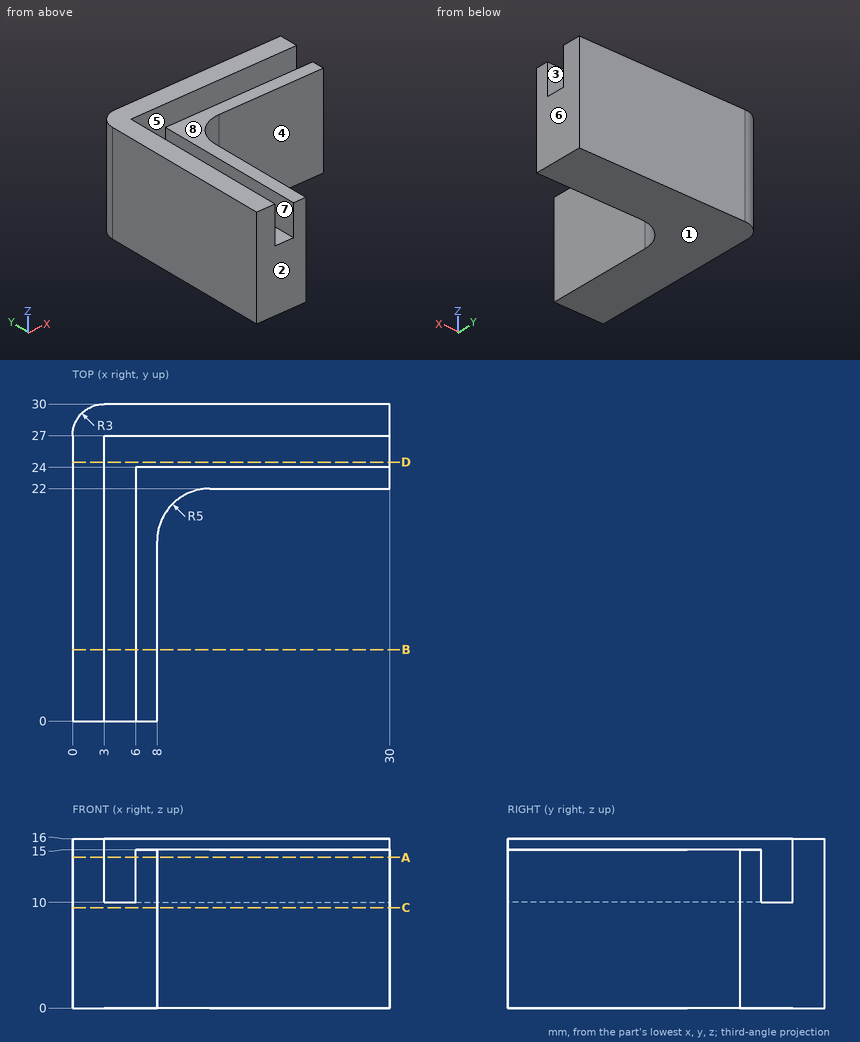
Verification items for this drawing (mm, ordinates from the low corner). A direction names the side the tool comes from. Coordinates: 2 decimals unless noted, no trailing zeros. Loops run counter-clockwise (first coordinate to the right, second up) from the corner with the lowest first, then second, coordinate; pieces in that order, holes last. Notation, with made-up numbers: (24.5, 57) - (41.5, 57) arc R22 cw to (41.5, 71) - close; hole circle Ø8 at (-31.75, 74). An arc over 180 degrees is marked (long way). One line per item, written item: value. Start each with the question number.
(1) Cross-section at D-D on y = 24.5. Enter the section's corners in (x, z).
(2) Cross-section at A-A on z = 14.25. Enter the section's corners in (x, y).
(3) Depth check by flat-ended pin: P1, Ø1.8, axis at y = 9, z = 12, coming from the +X side; P2, Ø4.5, axis at x = 24.5, z = 9, coming from the -Y side; P3, Ø1, axis at x = 9.5, y = 22, coming from the +Z side. Enter the tip coordinate at first touch or a pass-through.
(4) Tool access check on the marked faces 4, 5, 6, 7 and 8. Record the directions out of +Z, -Z, +X, -X, +Y, -Y that give a thin tool (end or side, any length) a straight path to the whole face; none if there is none.
(5) Mould release check, pull along Y, two halves, no side actions. Record for the marked faces 1, 2 and 3: released by +Y, released by -Y, zero draft, split by the parting line, or undercut.
(6) Cross-section at C-C on z = 9.5. Enter the section's corners in (x, y), plus the area to 3 significant figures.
(7) Cross-section at B-B on y = 6.75. Enter the section's corners in (x, z), plus the area to 3 significant figures.
(8) Material ranges on line 1 (Y direction, x = 17.25, z = 13); line 2 (X direction, y = 12, z = 14.5); line 3 (Y direction, x = 7.75, z = 14), recorded low to high. Write a range as [from, to].
Results below:
1. outline: (0, 0) - (30, 0) - (30, 10) - (3, 10) - (3, 16) - (0, 16) - close
2. outline: (0, 0) - (3, 0) - (3, 27) - (30, 27) - (30, 30) - (3, 30) arc R3 ccw to (0, 27) - close; (6, 0) - (8, 0) - (8, 17) arc R5 cw to (13, 22) - (30, 22) - (30, 24) - (6, 24) - close
3. P1: stops at x = 8
3. P2: stops at y = 22
3. P3: stops at z = 15
4. face 4: +Z, -Z, +X, -Y
4. face 5: +Z, +X
4. face 6: +Z, -Z, +X, +Y, -Y
4. face 7: +Z, -Y
4. face 8: +Z, +X, -Y
5. face 1: zero draft
5. face 2: released by -Y
5. face 3: undercut
6. outline: (0, 0) - (8, 0) - (8, 17) arc R5 cw to (13, 22) - (30, 22) - (30, 30) - (3, 30) arc R3 ccw to (0, 27) - close
6. area: 419 mm2
7. outline: (0, 0) - (8, 0) - (8, 15) - (6, 15) - (6, 10) - (3, 10) - (3, 16) - (0, 16) - close
7. area: 108 mm2
8. line 1: y = [22, 24], [27, 30]
8. line 2: x = [0, 3], [6, 8]
8. line 3: y = [0, 24], [27, 30]
